Source: CAD feature listing. Evaluate the final solid. Frame: model axes, mm. Round coordinates to 2 decimals unless told otherwise and drop trailing zeros. Order: outer loops, then holes, each group sorted by start corner. A loop starts at its lowest first (then second) coordinate and runs counter-clockwise, first axis right, second up. Notation, with made-up numbers: M -16,88.5 L 35,88.5 A19 cw 35,94.5 Z; hole C -8,54 d1. An arc over 180 degrees is marked long. Answer in a Markdown table with one row per item. Add a question column.
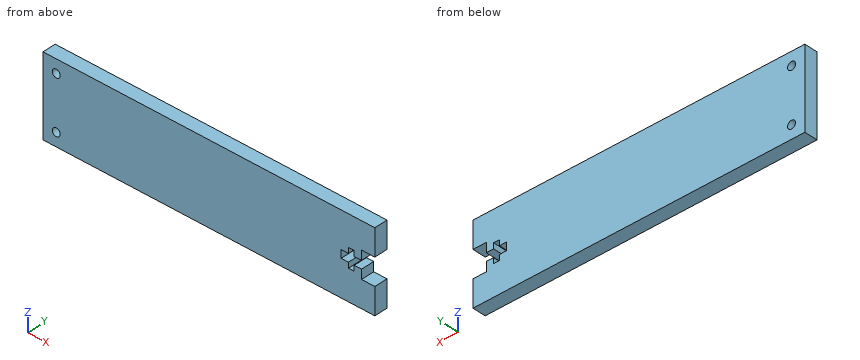
```python
from build123d import *

# Parameters (mm, degrees)
SKETCH1_W             = 158.75
SKETCH1_H             = 38.1
BOSS_EXTRUDE1_DEPTH   = 3.175
CUT_EXTRUDE1_REACH    = 83.876
F_6_CLEARANCE_HOLE1_D = 3.7973


with BuildPart() as part:
    # Sketch1 → Boss-Extrude1 (new, symmetric)
    with BuildSketch(Plane(origin=(0, 0, 0), x_dir=(1, 0, 0), z_dir=(0, 1, 0))):
        Rectangle(SKETCH1_W, SKETCH1_H)
    extrude(amount=BOSS_EXTRUDE1_DEPTH, both=True)

    # Sketch2 → Cut-Extrude1 (cut, up to next)
    with BuildSketch(Plane(origin=(0, 3.175, 0), x_dir=(1, 0, 0), z_dir=(0, 1, 0)), mode=Mode.PRIVATE) as cut_extrude1_sk1:
        Polygon((79.375, -6.35), (79.375, 6.35), (73.025, 6.35), (73.025, 1.89865), (69.524626, 1.89865), (69.524626, 4.504546622), (66.746374, 4.504546622), (66.746374, 1.89865), (63.246, 1.89865), (63.246, -1.89865), (66.746374, -1.89865), (66.746374, -4.504546622), (69.524626, -4.504546622), (69.524626, -1.89865), (73.025, -1.89865), (73.025, -6.35), align=None)
    cut_extrude1_tool1 = extrude(cut_extrude1_sk1.sketch, amount=-CUT_EXTRUDE1_REACH, mode=Mode.PRIVATE) & part.part
    add(cut_extrude1_tool1.solids().sort_by_distance((73.052853, 3.175, 0))[0], mode=Mode.SUBTRACT)

    # #6 Clearance Hole1 (through all)
    with Locations(Plane(origin=(0, 3.175, 0), x_dir=(1, 0, 0), z_dir=(0, 1, 0))):
        with Locations((-73.025, -12.7)):
            f_6_clearance_hole1 = Hole(F_6_CLEARANCE_HOLE1_D / 2)

    # Mirror1: #6 Clearance Hole1 across plane
    add(f_6_clearance_hole1.mirror(Plane.XY), mode=Mode.SUBTRACT)


solid = part.part
```
(1) Line query: line 1 (X direction, y = -1.25, z = 12.7) (3 decimals); line 2 (Z direction, x = -72, y = -2); line 3 (X direction, y = 2.25, z = -1.5) (3 decimals). Output: solid intervals per line, ascending. Write a range as from..to.
(2) Cut plane B-B (y = -2). Return loops of the section in (x, z) (3 decimals), and give its area (3 significant figures).
(3) Cut plane A-A (z = 12.7). Return loops of the section in (x, y) (3 decimals), and give its area (3 significant figures).
(4) Pin query (flat end, axial travel): pin 1 (2 mm diameter, centred on y = -1.5, z = 3.5, fed in from +X) (3 decimals); pin 2 (3 mm diameter, centred on x = -73.025, z = 12.7, fed in from +Y). Return the tip coordinate at first contact, or that it passes through.
Answer list:
| question | item | result |
|---|---|---|
| 1 | line 1 | -79.375..-74.924, -71.126..79.375 |
| 1 | line 2 | -19.05..-14.3, -11.1..11.1, 14.3..19.05 |
| 1 | line 3 | -79.375..63.246 |
| 2 | outline | M -79.375,-19.05 L 79.375,-19.05 L 79.375,-6.35 L 73.025,-6.35 L 73.025,-1.899 L 69.525,-1.899 L 69.525,-4.505 L 66.746,-4.505 L 66.746,-1.899 L 63.246,-1.899 L 63.246,1.899 L 66.746,1.899 L 66.746,4.505 L 69.525,4.505 L 69.525,1.899 L 73.025,1.899 L 73.025,6.35 L 79.375,6.35 L 79.375,19.05 L -79.375,19.05 Z; hole C -73.025,-12.7 d3.797; hole C -73.025,12.7 d3.797 |
| 2 | area | 5,890 mm² |
| 3 | outline | M -79.375,-3.175 L -74.924,-3.175 L -74.924,3.175 L -79.375,3.175 Z; M -71.126,-3.175 L 79.375,-3.175 L 79.375,3.175 L -71.126,3.175 Z |
| 3 | area | 984 mm² |
| 4 | pin 1 | x = 73.025 |
| 4 | pin 2 | through |
